```python
from build123d import *

# Parameters (mm, degrees)
SKETCH_1_R          = 43
SKETCH_1_R_2        = 9.5
SKETCH_1_R_3        = 3
EXTRUDE_1_DEPTH     = 12
CUT_EXTRUDE_1_DEPTH = 62.983868869


with BuildPart() as part:
    # 草图1 → 凸台-拉伸1 (new body)
    with BuildSketch(Plane.XY):
        Circle(SKETCH_1_R)
        Circle(SKETCH_1_R_2, mode=Mode.SUBTRACT)
        with Locations((0, -32)):
            Circle(SKETCH_1_R_3, mode=Mode.SUBTRACT)
        with Locations((-30.433808521, -9.88854382)):
            Circle(SKETCH_1_R_3, mode=Mode.SUBTRACT)
        with Locations((-18.809128073, 25.88854382)):
            Circle(SKETCH_1_R_3, mode=Mode.SUBTRACT)
        with Locations((18.809128073, 25.88854382)):
            Circle(SKETCH_1_R_3, mode=Mode.SUBTRACT)
        with Locations((30.433808521, -9.88854382)):
            Circle(SKETCH_1_R_3, mode=Mode.SUBTRACT)
    extrude(amount=EXTRUDE_1_DEPTH)

    # 草图2 → 切除-拉伸1 (cut, through all)
    with BuildSketch(Plane.XY.offset(12)):
        with BuildLine():
            ThreePointArc((-9.067424527, 9.315675631), (-12.343438055, 4.079158859), (-12.832801935, -2.078267189))
            ThreePointArc((-12.832801935, -2.078267189), (-21.37101475, -1.716157168), (-29.668995358, 0.32730058))
            ThreePointArc((-29.668995358, 0.32730058), (-32.591945887, 3.068256778), (-32.563681076, 7.075210954))
            ThreePointArc((-32.563681076, 7.075210954), (-31.298866838, 10.343394552), (-30.367210921, 13.721677599))
            ThreePointArc((-30.367210921, 13.721677599), (-28.002294185, 16.956434081), (-24.021676007, 17.415955129))
            ThreePointArc((-24.021676007, 17.415955129), (-16.140082755, 14.112519106), (-9.067424527, 9.315675631))
        make_face()
        with BuildLine():
            ThreePointArc((-5.942103436, 11.562500022), (-8.236169203, 19.794721108), (-8.856942422, 28.318032809))
            ThreePointArc((-8.856942422, 28.318032809), (-7.153379557, 31.944926002), (-3.33380537, 33.156261505))
            ThreePointArc((-3.33380537, 33.156261505), (0.165271032, 32.963275955), (3.666106648, 33.121165398))
            ThreePointArc((3.666106648, 33.121165398), (7.473342341, 31.871590651), (9.140451493, 28.227797607))
            ThreePointArc((9.140451493, 28.227797607), (8.434243395, 19.711139115), (6.057745738, 11.502335266))
            ThreePointArc((6.057745738, 11.502335266), (0.065178486, 12.999836605), (-5.942103436, 11.562500022))
        make_face()
        with BuildLine():
            ThreePointArc((30.503276045, 13.416485596), (31.401009953, 10.029030369), (32.632989436, 6.748328364))
            ThreePointArc((32.632989436, 6.748328364), (32.621073761, 2.741292217), (29.670785702, 0.02978322))
            ThreePointArc((29.670785702, 0.02978322), (21.352731843, -1.930365176), (12.811317288, -2.206841486))
            ThreePointArc((12.811317288, -2.206841486), (12.383720574, 3.955182012), (9.160380047, 9.224285197))
            ThreePointArc((9.160380047, 9.224285197), (16.280782246, 13.949967611), (24.195103905, 17.17420619))
            ThreePointArc((24.195103905, 17.17420619), (28.170914186, 16.674793259), (30.503276045, 13.416485596))
        make_face()
        with BuildLine():
            ThreePointArc((22.185866734, -24.864417397), (19.2416204, -26.764994313), (16.502189978, -28.950469101))
            ThreePointArc((16.502189978, -28.950469101), (12.687589993, -30.177378887), (9.197102544, -28.209390565))
            ThreePointArc((9.197102544, -28.209390565), (4.762470636, -20.904170405), (1.860083786, -12.866238312))
            ThreePointArc((1.860083786, -12.866238312), (7.588381736, -10.55539969), (11.603529654, -5.861578248))
            ThreePointArc((11.603529654, -5.861578248), (18.298245994, -11.173166982), (23.810338997, -17.703789654))
            ThreePointArc((23.810338997, -17.703789654), (24.563962018, -21.639337012), (22.185866734, -24.864417397))
        make_face()
        with BuildLine():
            ThreePointArc((-16.791656334, -28.783540658), (-19.509034547, -26.570706563), (-22.434075141, -24.640702259))
            ThreePointArc((-22.434075141, -24.640702259), (-24.77971191, -21.391938061), (-23.986663732, -17.464145391))
            ThreePointArc((-23.986663732, -17.464145391), (-18.409363119, -10.98912264), (-11.661722286, -5.744931098))
            ThreePointArc((-11.661722286, -5.744931098), (-7.693842741, -10.478777785), (-1.989004331, -12.846939782))
            ThreePointArc((-1.989004331, -12.846939782), (-4.971844287, -20.855364568), (-9.479505121, -28.115749926))
            ThreePointArc((-9.479505121, -28.115749926), (-12.989550761, -30.048639027), (-16.791656334, -28.783540658))
        make_face()
    extrude(amount=-CUT_EXTRUDE_1_DEPTH, mode=Mode.SUBTRACT)


solid = part.part
```
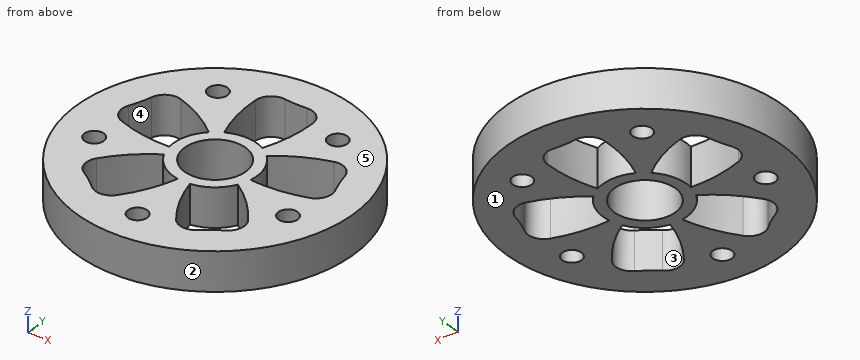
Part model, mm, in its own coordinate system. Face numbers are marked on the shaded views. A direction names the side the tool comes from. Round coordinates to 2 decimals unless told otherwise and drop trailing zeros. Loops run counter-clockwise (first coordinate to the right, second up) from the corner with the lowest first, then second, coordinate; pieces in that order, holes last.
1. Two-plate mould, pull along X, no slides. Class the marked faces 1, 2 and 3: pulls with the +X half, pulls with the -X half, needs draft (parallel to the pull), parting line crosses it, or undercut.
Solutions:
face 1: needs draft
face 2: parting line crosses it
face 3: undercut
2. Slice it at B-B (y = -32). Give the cut face in (x, z).
Solutions:
outline: (-28.72, 0) - (-3, 0) - (-3, 12) - (-28.72, 12) - close; (3, 0) - (28.72, 0) - (28.72, 12) - (3, 12) - close
3. 3-axis set-ups, long thin cutter, end or side, ignore diameter. For the marked faces 4 and 5: which of +Z, -Z, +X, -X, +Y, -Y reach the whole face in a straight line?
Solutions:
face 4: +Z, -Z
face 5: +Z, +X, -X, +Y, -Y
4. Flat gauge pins, fed straight in: pin 1 (3 mm diameter, centred on y = -34, z = 6.5, fed in from -X); pin 2 (2 mm diameter, centred on y = 22.5, z = 8, fed in from -X); pin 3 (5.5 mm diameter, centred on x = -30.43, y = -9.89, fed in from -Z); pin 4 (1.5 mm diameter, centred on y = -19, z = 2, fed in from -X). Where does each tip first touch, or does it go through?
Solutions:
pin 1: stops at x = -28.16
pin 2: stops at x = -37.24
pin 3: passes through
pin 4: stops at x = -38.94
5. Slice it at C-C (x = 19). Give the cut face in (y, z), and give its area (3 significant figures).
Solutions:
outline: (-38.57, 0) - (-26.94, 0) - (-26.94, 12) - (-38.57, 12) - close; (-11.87, 0) - (-2.18, 0) - (-2.18, 12) - (-11.87, 12) - close; (15.27, 0) - (22.89, 0) - (22.89, 12) - (15.27, 12) - close; (28.88, 0) - (38.57, 0) - (38.57, 12) - (28.88, 12) - close
area: 464 mm2
6. Slice it at A-A (y = -19). Give the cut face in (x, z).
Solutions:
outline: (-38.57, 0) - (-24.71, 0) - (-24.71, 12) - (-38.57, 12) - close; (-4.12, 0) - (3.91, 0) - (3.91, 12) - (-4.12, 12) - close; (24.45, 0) - (38.57, 0) - (38.57, 12) - (24.45, 12) - close
7. Slice it at D-D (x = 0). Give the cut face in (y, z), and give its area (3 significant figures).
Solutions:
outline: (-43, 0) - (-35, 0) - (-35, 12) - (-43, 12) - close; (-29, 0) - (-9.5, 0) - (-9.5, 12) - (-29, 12) - close; (9.5, 0) - (13, 0) - (13, 12) - (9.5, 12) - close; (32.96, 0) - (43, 0) - (43, 12) - (32.96, 12) - close
area: 492 mm2
8. Drill centre lines: line 1 along Y through (x, z) = (0, 4.5); line 2 along X through (y, z) = (-24, 8); line 3 along X through (y, z) = (-27, 9.75). Where is each one in solid material? Low to high.
Solutions:
line 1: y = -43 to -35, -29 to -9.5, 9.5 to 13, 32.96 to 43
line 2: x = -35.68 to -23.29, -6.68 to 6.4, 23.29 to 35.68
line 3: x = -33.47 to -18.94, -8.65 to 8.32, 18.92 to 33.47
